Source: three-view drawing plus pictorial views. Frame: mm from the lowest corner of the part. Give positions to 0.01 mm unless a question says otherwise; leave off trailing zeros. Loops run counter-clockwise (first coordinate to the right, second up) from the corner with the lowest first, then second, coordinate; pieces in that order, holes last.
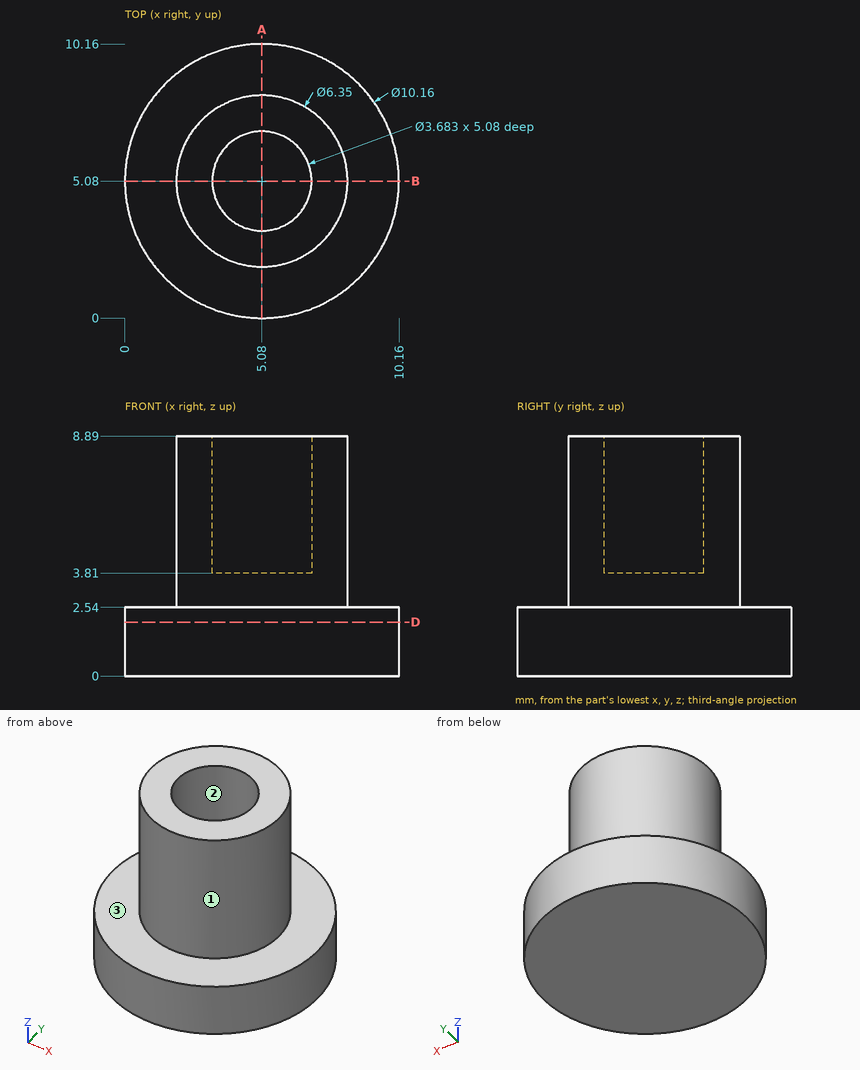
(1) Cut plane D-D (z = 2). Return the cut outline in (x, y), and give its area (3 significant figures).
Values follow:
outline: circle Ø10.16 at (5.08, 5.08)
area: 81.1 mm2
(2) Pin query (flat end, axial travel): pin 1 Ø6 at (x, y) = (5.08, 5.08) entering from +Z; pin 2 Ø1 at (x, z) = (8.5, 4) entering from +Y; pin 3 Ø1 at (y, z) = (8.5, 1.5) entering from -X. Return the tip coordinate at first contact, or that it passes through.
Values follow:
pin 1: stops at z = 8.89
pin 2: stops at y = 6.33
pin 3: stops at x = 0.92
(3) Mould query, pull axis Y, two halves, no side actions, for the marked faces 1, 2 and 3. Classes: +Y half, -Y half, draft (parallel to the pull), parting line (faces both ways), or undercut.
Values follow:
face 1: parting line
face 2: undercut
face 3: draft
(4) Cut plane A-A (x = 5.08). Return the cut outline in (y, z) (1 decimal).
Values follow:
outline: (0, 0) - (10.2, 0) - (10.2, 2.5) - (8.3, 2.5) - (8.3, 8.9) - (6.9, 8.9) - (6.9, 3.8) - (3.2, 3.8) - (3.2, 8.9) - (1.9, 8.9) - (1.9, 2.5) - (0, 2.5) - close
(5) Ray query, probe 1 along X at (y, z) = (5, 6.5); probe 2 along Y at (x, z) = (5.08, 7.1) (1 decimal); probe 3 along X at (y, z) = (6, 6.5). Return the intervals inside material, ascending.
Values follow:
probe 1: x = 1.91 to 3.24, 6.92 to 8.25
probe 2: y = 1.9 to 3.2, 6.9 to 8.3
probe 3: x = 2.04 to 3.48, 6.68 to 8.12
